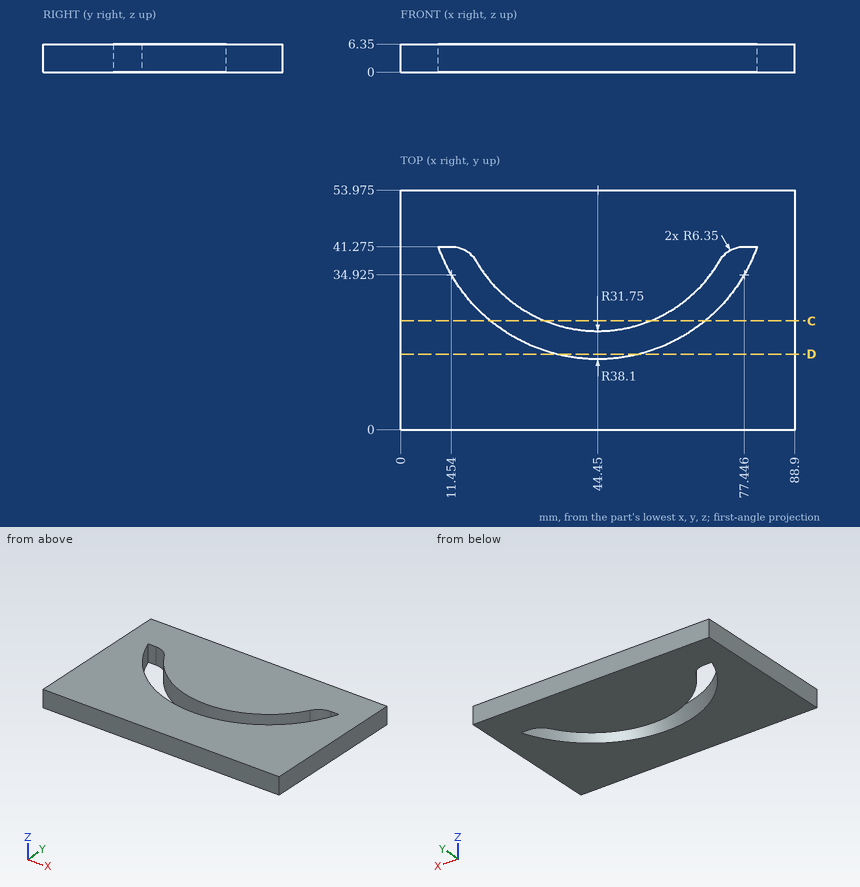
Study the drawing (mm; zero at the part's minimum x, y, z) and answer. Give positions to 0.01 mm unless a question says otherwise; leave off trailing zeros. Loops run counter-clockwise (first coordinate to the right, second up) from the corner with the lowest first, then second, coordinate; pieces in that order, holes last. Notation, with made-up numbers: M 48.25,-21 L 58.25,-21 A21 cw 58.25,17 Z; hole C 11,-33.75 d5. An arc over 180 degrees is marked long. Use CSV: the item, a comma, the result in double quotes.
1) Consider L1, parallel to Y at x = 69, z = 3.75 (1 decimal); L2, parallel to Y at x = 26, z = 5.25 (1 decimal); L3, parallel to X at y = 38, z = 2.25. Determine where each line is inside the solid, lowest interval first.
Answer:
L1,"0 to 24.8, 33.8 to 54"
L2,"0 to 20.6, 28.1 to 54"
L3,"0 to 9.86, 17.01 to 71.89, 79.04 to 88.9"
2) Given P1, Ø8, axis at x = 67.5, y = 18, coming from the -Z side, flat-ended and moving along its own axis, determine where the tip first touches the part or whether it passes through.
Answer:
P1,"z = 0"
3) Find section D-D on y = 17. Write down the section's boundary in (x, z).
Answer:
outline,"M 0,0 L 35.26,0 L 35.26,6.35 L 0,6.35 Z; M 53.64,0 L 88.9,0 L 88.9,6.35 L 53.64,6.35 Z"
4) Find section C-C on y = 24.5. Write down the section's boundary in (x, z), plus the area to 3 significant figures.
Answer:
outline,"M 0,0 L 20.31,0 L 20.31,6.35 L 0,6.35 Z; M 32.65,0 L 56.25,0 L 56.25,6.35 L 32.65,6.35 Z; M 68.59,0 L 88.9,0 L 88.9,6.35 L 68.59,6.35 Z"
area,"408 mm^2"
